Check sheet for the modelled part. Datum: model origin and axes. Units: mm. Round coordinates to 2 decimals unless told otherwise and drop trailing zeros. Put each result on its own line as item: value.
```python
from build123d import *

# Parameters (mm, degrees)
F0_R     = 4.1275
F0_R_2   = 2.5404111094
F0_R_3   = 1.5875
F0_R_4   = 4.7625
F1_DEPTH = 3.175


with BuildPart() as f1:
    # F0 (on Front) → F1 (new body)
    with BuildSketch(Plane.XZ):
        with BuildLine():
            ThreePointArc((-5.6526899501, 42.4243148479), (-10.2163375942, 38.7378035599), (-16.0377128052, 39.465014636))
            add(Edge.make_bspline(
                [(-16.0377128052, 39.465014636), (-19.3590733847, 41.2787515205), (-25.937027446, 44.8708571108), (-26.0510704547, 37.5423596471), (-26.1075305205, 33.9141894214)],
                knots=[0, 0, 0, 0, 0.5049230427, 1, 1, 1, 1], degree=3))
            ThreePointArc((-26.1075305205, 33.9141894214), (-28.2165096701, 28.4397531725), (-33.6215740259, 26.1588488329))
            add(Edge.make_bspline(
                [(-33.6215740259, 26.1588488329), (-37.4048251051, 26.0689107609), (-44.8975532223, 25.8907884246), (-41.3320686331, 19.487101945), (-39.5668793715, 16.3167843274)],
                knots=[0, 0, 0, 0, 0.5049230427, 1, 1, 1, 1], degree=3))
            ThreePointArc((-39.5668793715, 16.3167843274), (-38.6560907667, 10.5212938897), (-42.1965616381, 5.8434406101))
            add(Edge.make_bspline(
                [(-42.1965616381, 5.8434406101), (-45.4279841456, 3.8739264153), (-51.8278158705, -0.0266961114), (-45.5381723997, -3.789708986), (-42.4243148479, -5.6526899501)],
                knots=[0, 0, 0, 0, 0.5049230427, 1, 1, 1, 1], degree=3))
            ThreePointArc((-42.4243148479, -5.6526899501), (-38.7378035599, -10.2163375942), (-39.465014636, -16.0377128052))
            add(Edge.make_bspline(
                [(-39.465014636, -16.0377128052), (-41.2787515205, -19.3590733847), (-44.8708571108, -25.937027446), (-37.5423596471, -26.0510704547), (-33.9141894214, -26.1075305205)],
                knots=[0, 0, 0, 0, 0.5049230427, 1, 1, 1, 1], degree=3))
            ThreePointArc((-33.9141894214, -26.1075305205), (-28.4397531725, -28.2165096701), (-26.1588488329, -33.6215740259))
            add(Edge.make_bspline(
                [(-26.1588488329, -33.6215740259), (-26.0689107609, -37.4048251051), (-25.8907884246, -44.8975532223), (-19.487101945, -41.3320686331), (-16.3167843274, -39.5668793715)],
                knots=[0, 0, 0, 0, 0.5049230427, 1, 1, 1, 1], degree=3))
            ThreePointArc((-16.3167843274, -39.5668793715), (-10.5212938897, -38.6560907667), (-5.8434406101, -42.1965616381))
            add(Edge.make_bspline(
                [(-5.8434406101, -42.1965616381), (-3.8739264153, -45.4279841456), (0.0266961114, -51.8278158705), (3.789708986, -45.5381723997), (5.6526899501, -42.4243148479)],
                knots=[0, 0, 0, 0, 0.5049230427, 1, 1, 1, 1], degree=3))
            ThreePointArc((5.6526899501, -42.4243148479), (10.2163375942, -38.7378035599), (16.0377128052, -39.465014636))
            add(Edge.make_bspline(
                [(16.0377128052, -39.465014636), (19.3590733847, -41.2787515205), (25.937027446, -44.8708571108), (26.0510704547, -37.5423596471), (26.1075305205, -33.9141894214)],
                knots=[0, 0, 0, 0, 0.5049230427, 1, 1, 1, 1], degree=3))
            ThreePointArc((26.1075305205, -33.9141894214), (28.2165096701, -28.4397531725), (33.6215740259, -26.1588488329))
            add(Edge.make_bspline(
                [(33.6215740259, -26.1588488329), (37.4048251051, -26.0689107609), (44.8975532223, -25.8907884246), (41.3320686331, -19.487101945), (39.5668793715, -16.3167843274)],
                knots=[0, 0, 0, 0, 0.5049230427, 1, 1, 1, 1], degree=3))
            ThreePointArc((39.5668793715, -16.3167843274), (38.6560907667, -10.5212938897), (42.1965616381, -5.8434406101))
            add(Edge.make_bspline(
                [(42.4243148479, 5.6526899501), (45.5381723997, 3.789708986), (51.8278158705, 0.0266961114), (45.4279841456, -3.8739264153), (42.1965616381, -5.8434406101)],
                knots=[0, 0, 0, 0, 0.4950769573, 1, 1, 1, 1], degree=3))
            ThreePointArc((42.4243148479, 5.6526899501), (38.7378035599, 10.2163375942), (39.465014636, 16.0377128052))
            add(Edge.make_bspline(
                [(33.9141894214, 26.1075305205), (37.5423596471, 26.0510704547), (44.8708571108, 25.937027446), (41.2787515205, 19.3590733847), (39.465014636, 16.0377128052)],
                knots=[0, 0, 0, 0, 0.4950769573, 1, 1, 1, 1], degree=3))
            ThreePointArc((33.9141894214, 26.1075305205), (28.4397531725, 28.2165096701), (26.1588488329, 33.6215740259))
            add(Edge.make_bspline(
                [(16.3167843274, 39.5668793715), (19.487101945, 41.3320686331), (25.8907884246, 44.8975532223), (26.0689107609, 37.4048251051), (26.1588488329, 33.6215740259)],
                knots=[0, 0, 0, 0, 0.4950769573, 1, 1, 1, 1], degree=3))
            ThreePointArc((16.3167843274, 39.5668793715), (10.5212938897, 38.6560907667), (5.8434406101, 42.1965616381))
            add(Edge.make_bspline(
                [(-5.6526899501, 42.4243148479), (-3.7759205366, 45.5406430422), (0.0104416401, 51.8278017738), (3.8879032615, 45.4254752545), (5.8434406101, 42.1965616381)],
                knots=[0, 0, 0, 0, 0.4956655824, 1, 1, 1, 1], degree=3))
        make_face()
        with Locations((-16.9599252474, -29.3697753454)):
            Circle(F0_R, mode=Mode.SUBTRACT)
        with Locations((-29.396216652, -16.9902134209)):
            Circle(F0_R, mode=Mode.SUBTRACT)
        with Locations((-33.9765799749, -0.0510526042)):
            Circle(F0_R, mode=Mode.SUBTRACT)
        with Locations((-15.4859397151, -15.9911519154)):
            Circle(F0_R_2, mode=Mode.SUBTRACT)
        with Locations((-5.4156412371, -21.591713652)):
            Circle(F0_R_2, mode=Mode.SUBTRACT)
        with Locations((-21.4067931524, -6.1057739369)):
            Circle(F0_R_2, mode=Mode.SUBTRACT)
        with Locations((-7.1021895773, -12.2543237497)):
            Circle(F0_R_3, mode=Mode.SUBTRACT)
        with Locations((-12.3407943156, -7.0539097078)):
            Circle(F0_R_3, mode=Mode.SUBTRACT)
        with Locations((0, -33.8726447575)):
            Circle(F0_R, mode=Mode.SUBTRACT)
        with Locations((16.9391608166, -29.2922814346)):
            Circle(F0_R, mode=Mode.SUBTRACT)
        with Locations((6.1057739369, -21.4067931524)):
            Circle(F0_R_2, mode=Mode.SUBTRACT)
        with Locations((0.0347822273, -14.1387120511)):
            Circle(F0_R_3, mode=Mode.SUBTRACT)
        with Locations((15.9911519154, -15.4859397151)):
            Circle(F0_R_2, mode=Mode.SUBTRACT)
        with Locations((7.1577752669, -12.2021542883)):
            Circle(F0_R_3, mode=Mode.SUBTRACT)
        with Locations((12.3581893089, -6.9635495501)):
            Circle(F0_R_3, mode=Mode.SUBTRACT)
        with Locations((21.591713652, -5.4156412371)):
            Circle(F0_R_2, mode=Mode.SUBTRACT)
        with Locations((29.3187227412, -16.8559900301)):
            Circle(F0_R, mode=Mode.SUBTRACT)
        with Locations((-29.4737105627, 16.9088726432)):
            Circle(F0_R, mode=Mode.SUBTRACT)
        with Locations((-21.591713652, 5.4156412371)):
            Circle(F0_R_2, mode=Mode.SUBTRACT)
        with Locations((-14.2773520783, 0.0690833318)):
            Circle(F0_R_3, mode=Mode.SUBTRACT)
        with Locations((-3.8251928054, 0)):
            Circle(F0_R_4, mode=Mode.SUBTRACT)
        with Locations((-12.3929637769, 7.2060551365)):
            Circle(F0_R_3, mode=Mode.SUBTRACT)
        with Locations((-7.192549735, 12.4446598747)):
            Circle(F0_R_3, mode=Mode.SUBTRACT)
        with Locations((-15.9911519154, 15.4859397151)):
            Circle(F0_R_2, mode=Mode.SUBTRACT)
        with Locations((-0.0695566954, 14.3812176375)):
            Circle(F0_R_3, mode=Mode.SUBTRACT)
        with Locations((-6.1057739369, 21.4067931524)):
            Circle(F0_R_2, mode=Mode.SUBTRACT)
        with Locations((-17.0941486382, 29.3451640477)):
            Circle(F0_R, mode=Mode.SUBTRACT)
        with Locations((-0.1549878216, 33.9255273706)):
            Circle(F0_R, mode=Mode.SUBTRACT)
        with Locations((12.3060198475, 7.2964152942)):
            Circle(F0_R_3, mode=Mode.SUBTRACT)
        with Locations((7.0674151092, 12.4968293361)):
            Circle(F0_R_3, mode=Mode.SUBTRACT)
        with Locations((14.2425776102, 0.1734222545)):
            Circle(F0_R_3, mode=Mode.SUBTRACT)
        with Locations((21.4067931524, 6.1057739369)):
            Circle(F0_R_2, mode=Mode.SUBTRACT)
        with Locations((5.4156412371, 21.591713652)):
            Circle(F0_R_2, mode=Mode.SUBTRACT)
        with Locations((15.4859397151, 15.9911519154)):
            Circle(F0_R_2, mode=Mode.SUBTRACT)
        with Locations((33.8215921533, 0.1039352173)):
            Circle(F0_R, mode=Mode.SUBTRACT)
        with Locations((29.2412288304, 17.043096034)):
            Circle(F0_R, mode=Mode.SUBTRACT)
        with Locations((16.8049374259, 29.4226579585)):
            Circle(F0_R, mode=Mode.SUBTRACT)
    extrude(amount=F1_DEPTH)


solid = f1.part
```
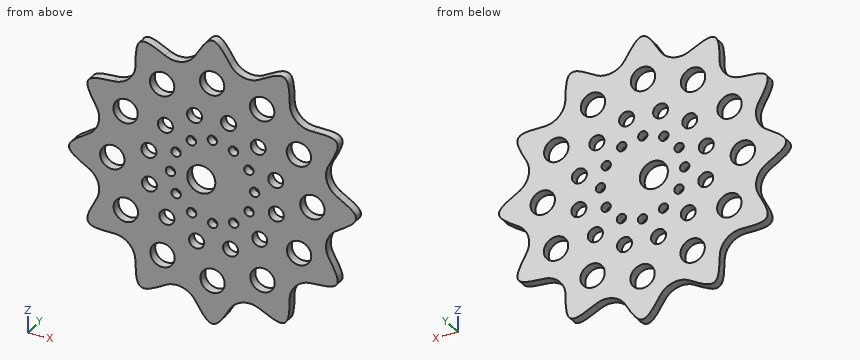
1. Scan lines: probe 1 along X at (y, z) = (-2, 23.5); probe 2 along X at (y, z) = (-2.8, -8); probe 3 along X at (y, z) = (-1.2, -41.5). Record each from-to range of solid material in increasing order.
Computed values:
probe 1: x = -42.4 to -7.55, -4.67 to 3.74, 7.09 to 42.38
probe 2: x = -39.79 to -23.1, -19.71 to -13.62, -11.07 to 11.16, 13.56 to 39.82
probe 3: x = -24.98 to -20, -6.3 to 6.24, 20 to 25.01
2. Depth check by flat-ended pin: pin 1 Ø4.5 at (x, z) = (21.59, -5.42) entering from -Y; pin 2 Ø6 at (x, z) = (20, 18) entering from +Y. Enter the tip coordinate at first touch or a pass-through.
Computed values:
pin 1: passes through
pin 2: stops at y = 0
3. Cross-section at A-A (y = -1.35). Count the separate pieces of the cut face and the enclosed holes in it, then the cut area to 3 significant figures.
Computed values:
separate pieces: 1
enclosed holes: 37
area: 4,950 mm2
